For this review, take the finished solid that the model builds, in its own axes (mm). A direction names the side the tool comes from. Give positions to 0.01 mm unless a question says otherwise; leave off trailing zeros. Order: outer loops, then holes, each group sorted by start corner. A loop starts at its lowest first (then second) coordinate and runs counter-clockwise, first axis right, second up.
Item 1: For P1, Ø11, axis at x = 43, z = 32.5, coming from the +Y side; P2, Ø0.8, axis at x = -15.5, y = 17.5, coming from the +Z side; P3, Ø6.5, axis at x = 43, z = -32.5, coming from the +Y side, all flat-tipped, find the tip position at first contact; note any pin that passes through.
Item 2: The part is to be moulded in two halves that separate along Y. For faces 6 (the flat face through (-43, -1, 32)), 7 (the flat face through (-40, -19, 6)), 8 (the flat face through (-45, 4, -29)), say which applies: released by +Y, released by -Y, zero draft, split by the parting line, or undercut.
Item 3: Consider section B-B (x = 17). Give the boundary of the cut face in (y, z).
Item 4: For probe 1 along Z at (x, y) = (43, 3); probe 2 along Y at (x, z) = (-40, -4); probe 3 along X at (y, z) = (3, -32), list the stretches that pass through material, from the lowest coordinate up.
Item 5: Consider section C-C (z = 22.5). Give the boundary of the cut face in (x, y).
Item 6: Machinability: for faces 1 (the cylindrical face through (37.098, -2.521, -36.263)), 2 (the flat face through (-49, 0, -38)), 3 (the flat face through (-25.46, 17.49, 2.5)), 4 (the cylindrical face through (39.53, 1.97, 32.96)), 5 (the cylindrical face through (-26.4, 8.4, -26.5)), which of the approach directions +Z, -Z, +X, -X, +Y, -Y give a long, thin tool a straight path to every point of the face, cutting with its end or side? Answer none if there is none.
Item 7: Consider section A-A (y = 1.5). Give the number of separate pieces and of enclosed holes in the cut face, plus the area to 3 significant figures.
Item 8: Consider section D-D (y = 12.5). Give the boundary of the cut face in (x, z).
```python
from build123d import *

# Parameters (mm, degrees)
ESQUISSE4_W             = 100
ESQUISSE4_H             = 79
BOSS_EXTRU_3_DEPTH      = 1
BOSS_EXTRU_4_DEPTH      = 4
BOSS_EXTRU_4_DEPTH_BACK = 4
ESQUISSE1_R             = 7
ESQUISSE1_R_2           = 3.5
ESQUISSE6_R             = 11.5
BOSS_EXTRU_5_DEPTH      = 17
BOSS_EXTRU_6_DEPTH      = 1
ESQUISSE8_W             = 65
ESQUISSE8_H             = 37
ENL_V_MAT_EXTRU_1_DEPTH = 1
ESQUISSE9_R             = 1
BOSS_EXTRU_7_DEPTH      = 18
ESQUISSE10_R            = 14.5
BOSS_EXTRU_8_DEPTH      = 2
ESQUISSE11_R            = 7.5
BOSS_EXTRU_9_DEPTH      = 4
CONG_1_R                = 3


with BuildPart() as part:
    # Esquisse4 → Boss.-Extru.3 (new body)
    with BuildSketch(Plane(origin=(0, 0, 0), x_dir=(1, 0, 0), z_dir=(0, 1, 0))):
        Rectangle(ESQUISSE4_W, ESQUISSE4_H)
    extrude(amount=-BOSS_EXTRU_3_DEPTH)

    # Esquisse1 → Boss.-Extru.4 (add, two sides: drawn at the far end of the back side and taken through both)
    # profile 1 of 4: a face of its own
    with BuildSketch(Plane(origin=(0, 0, 0), x_dir=(1, 0, 0), z_dir=(0, 1, 0)).offset(-BOSS_EXTRU_4_DEPTH_BACK)):
        with Locations(Location((43, 32.5, 0), (0, 0, 90))):
            Circle(ESQUISSE1_R)
        with Locations(Location((43, 32.5, 0), (0, 0, 90))):
            Circle(ESQUISSE1_R_2, mode=Mode.SUBTRACT)
    # profile 2 of 4: a face of its own
    with BuildSketch(Plane(origin=(0, 0, 0), x_dir=(1, 0, 0), z_dir=(0, 1, 0)).offset(-BOSS_EXTRU_4_DEPTH_BACK)):
        with Locations(Location((-43, 32.5, 0), (0, 0, 90))):
            Circle(ESQUISSE1_R)
        with Locations(Location((-43, 32.5, 0), (0, 0, 90))):
            Circle(ESQUISSE1_R_2, mode=Mode.SUBTRACT)
    # profile 3 of 4: a face of its own
    with BuildSketch(Plane(origin=(0, 0, 0), x_dir=(1, 0, 0), z_dir=(0, 1, 0)).offset(-BOSS_EXTRU_4_DEPTH_BACK)):
        with Locations(Location((-43, -32.5, 0), (0, 0, 270))):
            Circle(ESQUISSE1_R)
        with Locations(Location((-43, -32.5, 0), (0, 0, 90))):
            Circle(ESQUISSE1_R_2, mode=Mode.SUBTRACT)
    # profile 4 of 4: a face of its own
    with BuildSketch(Plane(origin=(0, 0, 0), x_dir=(1, 0, 0), z_dir=(0, 1, 0)).offset(-BOSS_EXTRU_4_DEPTH_BACK)):
        with Locations(Location((43, -32.5, 0), (0, 0, 270))):
            Circle(ESQUISSE1_R)
        with Locations(Location((43, -32.5, 0), (0, 0, 90))):
            Circle(ESQUISSE1_R_2, mode=Mode.SUBTRACT)
    extrude(amount=BOSS_EXTRU_4_DEPTH + BOSS_EXTRU_4_DEPTH_BACK)

    # Esquisse6 → Boss.-Extru.5 (add)
    with BuildSketch(Plane(origin=(0, 0, 0), x_dir=(1, 0, 0), z_dir=(0, 1, 0))):
        with Locations(Location((-38.5, -9.5, 0), (0, 0, 180))):
            Circle(ESQUISSE6_R)
        with Locations(Location((-15, 28, 0), (0, 0, 90))):
            Circle(ESQUISSE6_R)
    extrude(amount=BOSS_EXTRU_5_DEPTH)

    # Esquisse7 → Boss.-Extru.6 (add)
    with BuildSketch(Plane(origin=(0, 17, 0), x_dir=(1, 0, 0), z_dir=(0, 1, 0))):
        Polygon((-38.143774149, -19.88751618), (-28.414215556, -15.025120102), (-28.414215556, -3.974879898), (-22.428299765, -0.98338823), (-22.428299765, 19.221027247), (-7.571700235, 19.221027247), (-7.571700235, 34.680148422), (-13.988712335, 34.680148422), (-15.667356388, 38.039082045), (-35.613243864, 38.039082045), (-35.613243864, 23.559466539), (-38.143774149, 23.559466539), (-38.143774149, 0), align=None)
    extrude(amount=BOSS_EXTRU_6_DEPTH)

    # Esquisse8 → Enl_v. mat.-Extru.1 (cut)
    with BuildSketch(Plane(origin=(0, 0, 0), x_dir=(1, 0, 0), z_dir=(0, 1, 0))):
        with Locations((5.5, -8)):
            Rectangle(ESQUISSE8_W, ESQUISSE8_H)
    extrude(amount=-ENL_V_MAT_EXTRU_1_DEPTH, mode=Mode.SUBTRACT)

    # Esquisse9 → Boss.-Extru.7 (add)
    with BuildSketch(Plane.XZ.offset(1)):
        with Locations(Location((-40, 9.5, 0), (0, 0, 270))):
            Circle(ESQUISSE9_R)
    extrude(amount=BOSS_EXTRU_7_DEPTH)

    # Esquisse10 → Boss.-Extru.8 (add)
    with BuildSketch(Plane.XZ.offset(19)):
        with Locations(Location((-40, 9.5, 0), (0, 0, 270))):
            Circle(ESQUISSE10_R)
    extrude(amount=BOSS_EXTRU_8_DEPTH)

    # Esquisse11 → Boss.-Extru.9 (add)
    with BuildSketch(Plane(origin=(0, -21, 0), x_dir=(-1, 0, 0), z_dir=(0, -1, 0))):
        with Locations(Location((40, -9.5, 0), (0, 0, 90))):
            Circle(ESQUISSE11_R)
    extrude(amount=BOSS_EXTRU_9_DEPTH)

    # Cong_1
    cong_1_edges = [part.edges().sort_by_distance(p)[0] for p in [
        (-40, -25, 17),
    ]]
    fillet(cong_1_edges, radius=CONG_1_R)


solid = part.part
```
Resolved:
1. P1: stops at y = 4
1. P2: stops at z = -19.22
1. P3: stops at y = 0
2. face 6: released by -Y
2. face 7: undercut
2. face 8: released by +Y
3. outline: (-1, -39.5) - (0, -39.5) - (0, -10.5) - (-1, -10.5) - close; (-1, 26.5) - (0, 26.5) - (0, 39.5) - (-1, 39.5) - close
4. probe 1: z = -39.5 to -36, -29 to -25.5, 25.5 to 29, 36 to 39.5
4. probe 2: y = -21 to -19, -1 to 0
4. probe 3: x = -49.98 to -46.46, -39.54 to -36.02, -25.78 to -4.22, 36.02 to 39.54, 46.46 to 49.98
5. outline: (-50, -1) - (-27, -1) - (-27, 0) - (-50, 0) - close; (-46.42, -21) - (-33.58, -21) - (-33.58, -19) - (-46.42, -19) - close; (38, -1) - (50, -1) - (50, 0) - (38, 0) - close
6. face 1: -Y
6. face 2: -Z, -X, +Y
6. face 3: +Z, +X, +Y
6. face 4: +Y
6. face 5: none
7. separate pieces: 6
7. enclosed holes: 4
7. area: 1,290 mm2
8. outline: circle Ø23 at (-38.5, 9.5); circle Ø23 at (-15, -28)
